Here's how the part is built. I have some questions about the finished solid (model axes, mm). A direction names the side the tool comes from. Coordinates: 2 decimals unless noted, no trailing zeros. Write each loop counter-clockwise with the first axis right and the second up, starting at its lowest first coordinate (ties: lowest second). Pieces come first, ordered by that corner, then holes. Notation, with made-up numbers: (-29, 72.25) -> (17, 72.25) arc R25 cw to (17, 91.25) -> close; hole circle Ø2 at (9, 41). An arc over 180 degrees is marked (long way). Put each result on its own line as item: value. Start each with the question number.
Item 1: I want a section at A-A, the plane x = 39. List the corners of the cut face in (y, z) for me, then the cut area to 3 significant figures.
Item 2: I want a section at D-D, the plane z = 12. List the corners of the cut face in (x, y) for me, then the cut area to 3 significant figures.
Item 3: I want a section at C-C, the plane y = -21.25. List the corners of the cut face in (x, z) for me.
Item 4: If we mould it in two halves opening along X, with no side actions, what happens to faces 1 (the face through (27, 0, 11)), 2 (the face through (21.643, -12.878, 34.533)), 3 (the face through (3.665, -12.878, 34.238)), 4 (the face through (14.08, -12.88, 31.6))? For each: released by +X, released by -X, zero draft, split by the parting line, or undercut.
Item 5: I need wall thicknesses on line 1 (Z direction, x = 12.7, y = -12.75); line 2 (X direction, y = -16.5, z = 25.4); line 3 (X direction, y = -9, z = 2). Which ranges of each line are inside material? Lowest first, please. Write a range as [from, to].
Item 6: On a 3-axis mill with a long thin cutter (end or side, diameter ignored), from which of +Z, -Z, +X, -X, +Y, -Y can I reach the whole of each face in a straight line? I mean faces 5 (the face through (69.85, -13, 6)), 6 (the face through (25.4, -13, 19)), 7 (the face through (48, -19.05, 6)). Say none if no direction works.
Item 7: I want a section at B-B, the plane z = 21.5. List the corners of the cut face in (x, y) for me.
Item 8: For pin 1 (10 mm diameter, centred on x = 12.7, z = 25.4, fed in from +Y), with a flat end and sliding along its axis, tell me the tip position at first contact or that it passes through.
from build123d import *

# Parameters (mm, degrees)
F1_DEPTH = 25.4
F3_DEPTH = 25.401
F5_DEPTH = 25.401
F7_DEPTH = 38.101


with BuildPart() as f1:
    # F0 (on Front) → F1 (new body)
    with BuildSketch(Plane.XZ):
        Polygon((0, 38.1), (0, 0), (69.85, 0), (69.85, 12.7), (25.4, 12.7), (25.4, 38.1), align=None)
    extrude(amount=F1_DEPTH)

    # F2 (on face) → F3 (cut, through all)
    with BuildSketch(Plane.XZ.offset(25.4)):
        with BuildLine():
            Line((6.35, 25.4), (19.05, 25.4))
            ThreePointArc((19.05, 25.4), (12.7, 31.75), (6.35, 25.4))
        make_face()
        with BuildLine():
            ThreePointArc((6.35, 25.4), (12.7, 19.05), (19.05, 25.4))
            Line((19.05, 25.4), (6.35, 25.4))
        make_face()
    extrude(amount=-F3_DEPTH, mode=Mode.SUBTRACT)

    # F4 (on face) → F5 (cut, through all)
    with BuildSketch(Plane.XZ.offset(25.4)):
        with BuildLine():
            ThreePointArc((0, 25.4), (3.7630086547, 34.3369913453), (12.7, 38.1))
            Line((12.7, 38.1), (0, 38.1))
            Line((0, 38.1), (0, 25.4))
        make_face()
        with BuildLine():
            ThreePointArc((13.0906473624, 38.1), (21.7385437163, 34.4385437163), (25.4, 25.7906473624))
            Line((25.4, 25.7906473624), (25.4, 38.1))
            Line((25.4, 38.1), (13.0906473624, 38.1))
        make_face()
    extrude(amount=-F5_DEPTH, mode=Mode.SUBTRACT)

    # F6 (on face) → F7 (cut, through all)
    with BuildSketch(Plane(origin=(0, 0, 0), x_dir=(1, 0, 0), z_dir=(0, 0, -1))):
        with BuildLine():
            Line((38.1, 6.35), (57.15, 6.35))
            ThreePointArc((57.15, 6.35), (61.6401280605, 8.2098719395), (63.5, 12.7))
            ThreePointArc((63.5, 12.7), (61.6401280605, 17.1901280605), (57.15, 19.05))
            Line((57.15, 19.05), (38.1, 19.05))
            ThreePointArc((38.1, 19.05), (33.6098719395, 17.1901280605), (31.75, 12.7))
            ThreePointArc((31.75, 12.7), (33.6098719395, 8.2098719395), (38.1, 6.35))
        make_face()
    extrude(amount=-F7_DEPTH, mode=Mode.SUBTRACT)


solid = f1.part
Calculated:
1. outline: (-25.4, 0) -> (-19.05, 0) -> (-19.05, 12.7) -> (-25.4, 12.7) -> close; (-6.35, 0) -> (0, 0) -> (0, 12.7) -> (-6.35, 12.7) -> close
1. area: 161 mm2
2. outline: (0, -25.4) -> (69.85, -25.4) -> (69.85, 0) -> (0, 0) -> close; hole (38.1, -19.05) -> (57.15, -19.05) arc R6.35 ccw to (57.15, -6.35) -> (38.1, -6.35) arc R6.35 ccw to start
2. area: 1,410 mm2
3. outline: (0, 0) -> (69.85, 0) -> (69.85, 12.7) -> (25.4, 12.7) -> (25.4, 25.79) arc R12.51 ccw to (13.09, 38.1) -> (12.7, 38.1) arc R12.85 ccw to (0, 25.4) -> close; hole circle Ø12.7 at (12.7, 25.4)
4. face 1: zero draft
4. face 2: released by +X
4. face 3: released by -X
4. face 4: undercut
5. line 1: z = [0, 19.05], [31.75, 38.1]
5. line 2: x = [0, 6.35], [19.05, 25.4]
5. line 3: x = [0, 32.94], [62.31, 69.85]
6. face 5: +Z, -Z, +X, +Y, -Y
6. face 6: +Z, +X, +Y, -Y
6. face 7: +Z, -Z
7. outline: (0, -25.4) -> (7.69, -25.4) -> (7.69, 0) -> (0, 0) -> close; (17.71, -25.4) -> (25.4, -25.4) -> (25.4, 0) -> (17.71, 0) -> close
8. pin 1: passes through
